from build123d import *

# Parameters (mm, degrees)
F0_W     = 5
F0_H     = 14.4
F1_DEPTH = 81.5
F2_DEPTH = 8
F3_DEPTH = 80
F4_W     = 8.4
F4_H     = 8.4
F5_DEPTH = 80


with BuildPart() as f1:
    # F0 (on Top) → F1 (new body)
    with BuildSketch(Plane.XY):
        Polygon((-4.2, -4.2), (-4.2, 4.2), (-4.2, 7.2), (-7.2, 7.2), (-7.2, -7.2), (-4.2, -7.2), align=None)
        with Locations((-9.7, 0)):
            Rectangle(F0_W, F0_H)
    extrude(amount=-F1_DEPTH)

    # F0 (on Top) → F2 (join)
    with BuildSketch(Plane.XY):
        Polygon((-4.2, 7.2), (-4.2, 4.2), (4.2, 4.2), (4.2, -4.2), (-4.2, -4.2), (-4.2, -7.2), (7.2, -7.2), (7.2, 7.2), align=None)
    extrude(amount=-F2_DEPTH)

    # F0 (on Top) → F3 (join)
    with BuildSketch(Plane.XY):
        with Locations((-9.7, 0)):
            Rectangle(F0_W, F0_H)
        Polygon((-4.2, -4.2), (-4.2, 4.2), (-4.2, 7.2), (-7.2, 7.2), (-7.2, -7.2), (-4.2, -7.2), align=None)
        Polygon((-4.2, 7.2), (-4.2, 4.2), (4.2, 4.2), (4.2, -4.2), (-4.2, -4.2), (-4.2, -7.2), (7.2, -7.2), (7.2, 7.2), align=None)
    extrude(amount=F3_DEPTH)

    # F4 (on face) → F5 (join)
    with BuildSketch(Plane.XY.offset(80)):
        Rectangle(F4_W, F4_H)
    extrude(amount=-F5_DEPTH)


solid = f1.part
Read the model definition and answer for the solid it produces. Units are mm, in the model's axes. A direction names the side the tool comes from. Give positions to 0.01 mm unless a question says otherwise; leave off trailing zeros. Write each loop counter-clockwise with the first axis right and the second up, starting at its lowest first coordinate (ties: lowest second). Pieces come first, ordered by that corner, then holes. Notation, with made-up numbers: (60.25, 31) - (81.25, 31) arc R25 cw to (81.25, 54) - close; hole circle Ø11 at (-33, 87). An arc over 180 degrees is marked (long way). Return JSON: item names as keys, results as strings.
Q1. A cutting plane is placed at A-A, the plane x = -1.25. Determine the outline of the cut face in (y, z).
Reply:
{"outline": "(-7.2, -8) - (-4.2, -8) - (-4.2, 0) - (4.2, 0) - (4.2, -8) - (7.2, -8) - (7.2, 80) - (-7.2, 80) - close"}
Q2. Consider line 1 along Z through (x, y) = (0.5, 1); line 2 along Z through (x, y) = (-3.75, -6.25); line 3 along X through (y, z) = (4, -12). Determine where each line is inside the solid, lowest interval first. Write a range as [from, to].
Reply:
{"line 1": "[0, 80]", "line 2": "[-8, 80]", "line 3": "[-12.2, -4.2]"}
Q3. For faces 4 (the face through (5, 0, -8)), 5 (the face through (0, -4.2, -4)), 6 (the face through (-12.2, 0, -2)), determine the directions among +Z, -Z, +X, -X, +Y, -Y from which every point of the face is accessible in a straight line to the end or side of a thin tool.
Reply:
{"face 4": "-Z, +X, +Y, -Y", "face 5": "-Z", "face 6": "+Z, -Z, -X, +Y, -Y"}
Q4. A cutting plane is placed at B-B, the plane y = 1.5. Determine the outline of the cut face in (x, z), and give its area (3 significant figures).
Reply:
{"outline": "(-12.2, -81.5) - (-4.2, -81.5) - (-4.2, 0) - (4.2, 0) - (4.2, -8) - (7.2, -8) - (7.2, 80) - (-12.2, 80) - close", "area": "2,230 mm²"}
Q5. Given P1, Ø2, axis at y = -5, z = -33, coming from the +X side; P2, Ø5.5, axis at x = -0.5, y = -3, coming from the -Z side; P3, Ø10, axis at x = -2, z = -17, coming from the -Y side; P4, Ø2.5, axis at x = -1.5, y = -0.5, coming from the -Z side, each flat-ended and moving along its own axis, determine where each tip first touches the part or whether it passes through.
Reply:
{"P1": "x = -4.2", "P2": "z = -8", "P3": "y = -7.2", "P4": "z = 0"}
Q6. A cutting plane is placed at C-C, the plane z = -24. Determine the outline of the cut face in (x, y).
Reply:
{"outline": "(-12.2, -7.2) - (-4.2, -7.2) - (-4.2, 7.2) - (-12.2, 7.2) - close"}
Q7. For a pull along Y with two mould halves and no side action, classify faces 1 (the face through (-5, -7.2, 16)), 2 (the face through (4.2, 0, -4)), 3 (the face through (-8, 0, -81.5)) as released by +Y, released by -Y, zero draft, split by the parting line, or undercut.
Reply:
{"face 1": "released by -Y", "face 2": "undercut", "face 3": "zero draft"}
